```python
from build123d import *

# Parameters (mm, degrees)
CYLINDER050_R     = 12.2
CYLINDER050_DEPTH = 2
CYLINDER003_R     = 0.5
CYLINDER003_DEPTH = 10
CYLINDER004_R     = 0.5
CYLINDER004_DEPTH = 10
BOX003_W          = 8
BOX003_H          = 2
BOX003_DEPTH      = 14
BOX004_W          = 10
BOX004_H          = 2
BOX004_DEPTH      = 4
PAD017_DEPTH      = 37
BOX002_W          = 8
BOX002_H          = 2
BOX002_DEPTH      = 14


with BuildPart() as cylinder050:
    # Cylinder050 → Cylinder050 (new body)
    with BuildSketch(Plane(origin=(25, -7, 21), x_dir=(1, 0, 0), z_dir=(0, 1, 0))):
        Circle(CYLINDER050_R)
    extrude(amount=CYLINDER050_DEPTH)


with BuildPart() as cylinder003:
    # Cylinder003 → Cylinder003 (new body)
    with BuildSketch(Plane(origin=(57, 0, 8), x_dir=(1, 0, 0), z_dir=(0, -1, 0))):
        Circle(CYLINDER003_R)
    extrude(amount=CYLINDER003_DEPTH)


with BuildPart() as fusion007:
    # Cylinder004 → Cylinder004 (new body)
    with BuildSketch(Plane(origin=(20, 0, 8), x_dir=(1, 0, 0), z_dir=(0, -1, 0))):
        Circle(CYLINDER004_R)
    extrude(amount=CYLINDER004_DEPTH)

    # Fusion007: union Cylinder003
    add(cylinder003.part)


with BuildPart() as cube003:
    # Box003 → Box003 (new body)
    with BuildSketch(Plane(origin=(16, -7, 0), x_dir=(1, 0, 0), z_dir=(0, 0, 1))):
        with Locations((4, 1)):
            Rectangle(BOX003_W, BOX003_H)
    extrude(amount=BOX003_DEPTH)


with BuildPart() as cube004:
    # Box004 → Box004 (new body)
    with BuildSketch(Plane(origin=(39, -7, 4), x_dir=(1, 0, 0), z_dir=(0, 0, 1))):
        with Locations((5, 1)):
            Rectangle(BOX004_W, BOX004_H)
    extrude(amount=BOX004_DEPTH)


with BuildPart() as cut002:
    # Sketch152 → Pad017 (new body)
    with BuildSketch(Plane.ZY):
        Polygon((-1, -5), (0, -13), (1.999611, -13), (1.999611, -7), (7.999909, -7), (7.999909, -5), align=None)
    extrude(amount=-PAD017_DEPTH)


with BuildPart() as cut002_1:
    # Body015 placement: moved
    add(cut002.part.moved(Location((16, 0, 0))))

    # Cut002: cut Cube004
    add(cube004.part, mode=Mode.SUBTRACT)


with BuildPart() as mountclip2:
    # Box002 → Box002 (new body)
    with BuildSketch(Plane(origin=(53, -7, 0), x_dir=(1, 0, 0), z_dir=(0, 0, 1))):
        with Locations((4, 1)):
            Rectangle(BOX002_W, BOX002_H)
    extrude(amount=BOX002_DEPTH)

    # Fusion006: union Cube003, Cut002
    add(cube003.part)
    add(cut002_1.part)

    # Cut003: cut Fusion007
    add(fusion007.part, mode=Mode.SUBTRACT)

    # Cut026: cut Cylinder050
    add(cylinder050.part, mode=Mode.SUBTRACT)


solid = mountclip2.part
```
Could you check a few things on this model? Use its own coordinates, in mm. A direction names the side the tool comes from. Coordinates: 2 decimals unless noted, no trailing zeros. Order: outer loops, then holes, each group sorted by start corner. A loop starts at its lowest first (then second) coordinate and runs counter-clockwise, first axis right, second up. Notation, with made-up numbers: M 49,33 L 108,33 A25 ccw 108,72 Z; hole C 44.25,82 d2. An arc over 180 degrees is marked long. Use one line per item in the form item = value. Start each with the question number.
1. Suppose I cut it at A-A on x = 57. Write out the boundary of the cut face in (y, z), then the cut area to 3 significant figures.
2. We'd pull the mould along Z, two halves only. Please class faces 4 (the flat face through (49, -6, 6)), 5 (the flat face through (51, -6, 8)), 6 (the flat face through (57, -6, 0)), 7 (the cylindrical face through (56.6, -6, 7.7)): +Z half, -Z half, draft (parallel to the pull), parting line (faces both ways), or undercut.
3. On a 3-axis mill with a long thin cutter (end or side, diameter ignored), from which of +Z, -Z, +X, -X, +Y, -Y can I reach the whole of each face in a straight line? I mean faces 1 (the flat face through (44, -6, 4)), 2 (the flat face through (61, -6, 7)), 3 (the flat face through (34, -10, 2)). Say none if no direction works.
4. Suppose I cut it at D-D on z = 0.75. Write out the boundary of the cut face in (x, y).
5. Please list where these lines run through material, in increasing order: line 1 (Z direction, x = 57, y = -6.5); line 2 (Z direction, x = 58, y = -5.25); line 3 (Y direction, x = 26, z = 2.25).
6. Suppose I cut it at B-B on z = 6.25. Write out the boundary of the cut face in (x, y).
7. For pin 1 (2 mm diameter, centred on x = 35, y = -6, fed in from +Z); pin 2 (1 mm diameter, centred on x = 46, y = -5.5, fed in from +Z); pin 3 (2 mm diameter, centred on x = 57, y = -6.5, fed in from -Z); pin 4 (4 mm diameter, centred on x = 45.5, z = 9, fed in from -Y), each with a flat end and sliding along its axis, tell me the tip position at first contact or that it passes through.
8. Suppose I cut it at C-C on x = 24.5. Write out the boundary of the cut face in (y, z), then the cut area to 3 significant figures.
Geometry says:
q1.outline = M -7,0 L -5,0 L -5,7.5 L -7,7.5 Z; M -7,8.5 L -5,8.5 L -5,14 L -7,14 Z
q1.area = 26.0 mm^2
q2.face_4 = draft
q2.face_5 = +Z half
q2.face_6 = -Z half
q2.face_7 = undercut
q3.face_1 = +Z, +Y, -Y
q3.face_2 = +Z, -Z, +X, +Y, -Y
q3.face_3 = +Z, +X, -X, -Y
q4.outline = M 16,-13 L 53,-13 L 53,-7 L 61,-7 L 61,-5 L 16,-5 Z
q5.line_1 = 0 to 7.5, 8.5 to 14
q5.line_2 = 0 to 14
q5.line_3 = -7 to -5
q6.outline = M 16,-7 L 39,-7 L 39,-5 L 16,-5 Z; M 49,-7 L 61,-7 L 61,-5 L 49,-5 Z
q7.pin_1 = 8
q7.pin_2 = 4
q7.pin_3 = 0
q7.pin_4 = through
q8.outline = M -13,0 L -5,-1 L -5,8 L -7,8 L -7,2 L -13,2 Z
q8.area = 32.0 mm^2
